Can you work these out from the model? Positions are in its coordinate system, mm. A direction names the side the tool comes from. Coordinates: 2 decimals unless noted, no trailing zeros. Loops run counter-clockwise (first coordinate to the right, second up) from the corner with the lowest first, then second, coordinate; pieces in that order, holes last. Notation, with made-up numbers: (73.25, -35) -> (114.25, -35) arc R27 ccw to (114.25, -4) -> close; hole circle Ø11 at (18, 71). An arc over 180 degrees is marked (long way). Put each result on its own line as item: value. Start each with the question number.
Item 1: For faces 1 (the flat face through (1, 0, 14.5)), 2 (the flat face through (41, 12.824, 1)), 3 (the flat face through (-0.75, 0, 11)), which set-ups out of +Z, -Z, +X, -X, +Y, -Y let a thin tool reach every point of the face, with its end or its side?
Item 2: We'd pull the mould along Z, two halves only. Please class faces 4 (the cylindrical face through (0.504, -3.842, 2.246)), 5 (the cylindrical face through (-2.265, -0.713, 7.923)), 6 (the flat face through (8, 5, 0)), 7 (the conical face through (2.257, -0.04, 14.215)): pulls with the +Z half, pulls with the -Z half, needs draft (parallel to the pull), parting line crosses it, or undercut.
Item 3: If we section it at A-A on z = 12: Please give me the cut outline in (x, y) (3 decimals), plus the area to 3 significant figures.
Item 4: Will these pins go through, and if not, where does the flat tip stop? P1, Ø20, axis at x = 21, y = -7, coming from the +Z side; P2, Ø8, axis at x = 19, z = 7, coming from the -Y side; P3, Ø4, axis at y = 1, z = 9.5, coming from the +X side (3 decimals); P4, Ø1.6, axis at x = 42, z = 1, coming from the -Y side.
Item 5: If we section it at B-B on y = 16: Please give me the cut outline in (x, z).
Item 6: If we section it at C-C on x = -8.5: Please give me the cut outline in (y, z), plus the area to 3 significant figures.
Item 7: Please list where these lines run through material, in increasing order: L1, parallel to X at y = 0, z = 8.5 (3 decimals); L2, parallel to Z at x = 31, y = 17.5; L3, parallel to Y at x = 42, z = 1.75. Write a range as from..to.
```python
from build123d import *

# Parameters (mm, degrees)
F1_DEPTH = 2
F5_DEPTH = 7


with BuildPart() as f1:
    # F0 (on Top) → F1 (new body)
    with BuildSketch(Plane.XY):
        with BuildLine():
            ThreePointArc((0, 20), (-14.1421356237, -14.1421356237), (20, 0))
            ThreePointArc((20, 0), (19.8801750957, 2.1860096442), (19.5221361835, 4.3458254488))
            ThreePointArc((19.5221361835, 4.3458254488), (12.5116643782, 15.6031488645), (0, 20))
        make_face()
        with BuildLine():
            ThreePointArc((0, 20), (12.5116643782, 15.6031488645), (19.5221361835, 4.3458254488))
            add(Edge.make_bspline(
                [(19.5221361835, 4.3458254488), (19.5522097075, 6.2540398569), (19.5931412655, 10.6298460328), (25.5746730025, 12.0320439415), (28.9447810501, 12.8235351294)],
                knots=[0, 0, 0, 0, 0.4357911991, 1, 1, 1, 1], degree=3))
            Line((28.9447810501, 12.8235351294), (53.3421300352, 12.8235351294))
            Line((53.3421300352, 12.8235351294), (53.3421300352, 20))
            Line((53.3421300352, 20), (0, 20))
        make_face()
    extrude(amount=F1_DEPTH)

    # F2 (on Front) → F3 (revolve)
    with BuildSketch(Plane.XZ):
        Polygon((-2.375, 0), (0, 0), (0, 14.5), (-2.1112329669, 14.5), (-2.625, 13.5), (-2.375, 13.5), (-2.375, 2.5), (-3.875, 2.5), (-3.875, 0), align=None)
    revolve(axis=Axis((0, 0, 6.1913983081), (0, 0, 1)))

    # F4 (on face) → F5 (cut)
    with BuildSketch(Plane.XY.offset(14.5)):
        with BuildLine():
            ThreePointArc((-0.75, 1.9735259412), (0, 2.1112329669), (0.75, 1.9735259412))
            Line((0.75, 1.9735259412), (0.75, 4.4615390464))
            Line((0.75, 4.4615390464), (-0.75, 4.4615390464))
            Line((-0.75, 4.4615390464), (-0.75, 1.9735259412))
        make_face()
        with BuildLine():
            ThreePointArc((-0.75, -1.9735259412), (0, -2.1112329669), (0.75, -1.9735259412))
            Line((0.75, -1.9735259412), (0.75, 1.9735259412))
            ThreePointArc((0.75, 1.9735259412), (0, 2.1112329669), (-0.75, 1.9735259412))
            Line((-0.75, 1.9735259412), (-0.75, -1.9735259412))
        make_face()
        with BuildLine():
            Line((-0.75, -4.4615390464), (0.75, -4.4615390464))
            Line((0.75, -4.4615390464), (0.75, -1.9735259412))
            ThreePointArc((0.75, -1.9735259412), (0, -2.1112329669), (-0.75, -1.9735259412))
            Line((-0.75, -1.9735259412), (-0.75, -4.4615390464))
        make_face()
    extrude(amount=-F5_DEPTH, mode=Mode.SUBTRACT)


solid = f1.part
```
Solutions:
1. face 1: +Z, +X, -X, +Y, -Y
1. face 2: +Z, -Z, +X, -Y
1. face 3: +Z, +Y, -Y
2. face 4: needs draft
2. face 5: undercut
2. face 6: pulls with the -Z half
2. face 7: pulls with the +Z half
3. outline: (-0.75, -2.253) -> (-0.75, 2.253) arc R2.375 ccw to start; (0.75, -2.253) arc R2.375 ccw to (0.75, 2.253) -> close
3. area: 10.7 mm^2
4. P1: z = 2
4. P2: through
4. P3: x = 2.375
4. P4: y = 12.82
5. outline: (-12, 0) -> (53.34, 0) -> (53.34, 2) -> (-12, 2) -> close
6. outline: (-18.1, 0) -> (18.1, 0) -> (18.1, 2) -> (-18.1, 2) -> close
6. area: 72.4 mm^2
7. L1: -2.375..-0.75, 0.75..2.375
7. L2: 0..2
7. L3: 12.82..20
